from build123d import *

# Parameters (mm, degrees)
F1_DEPTH = 12.7
F3_DEPTH = 12.701
F4_R     = 5.08
F5_DEPTH = 25.4


with BuildPart() as f1:
    # F0 (on Top) → F1 (new body)
    with BuildSketch(Plane.XY):
        Polygon((349.925731, -349.925731), (494.869714, 0), (349.925731, 349.925731), (0, -494.869714), align=None)
    extrude(amount=F1_DEPTH)

    # F2 (on face) → F3 (cut, through all)
    with BuildSketch(Plane.XY.offset(12.7)):
        with BuildLine():
            ThreePointArc((43.288021, -466.629443), (44.712917, -465.460061), (45.248001, -463.696126))
            ThreePointArc((45.248001, -463.696126), (39.433085, -461.93219), (43.288021, -466.629443))
        make_face()
        with BuildLine():
            ThreePointArc((299.347591, -360.566096), (300.772487, -359.396714), (301.307571, -357.632779))
            ThreePointArc((301.307571, -357.632779), (295.492655, -355.868843), (299.347591, -360.566096))
        make_face()
        with BuildLine():
            ThreePointArc((360.566096, -299.347591), (360.746772, -298.751982), (360.807779, -298.132571))
            ThreePointArc((360.807779, -298.132571), (358.252191, -295.018577), (354.699461, -296.917551))
            Line((354.699461, -296.917551), (357.632779, -298.132571))
            Line((357.632779, -298.132571), (360.566096, -299.347591))
        make_face()
        with BuildLine():
            Line((357.632779, -298.132571), (354.699461, -296.917551))
            ThreePointArc((354.699461, -296.917551), (356.417759, -301.065888), (360.566096, -299.347591))
            Line((360.566096, -299.347591), (357.632779, -298.132571))
        make_face()
        with BuildLine():
            ThreePointArc((466.629443, -43.288021), (466.810119, -42.692412), (466.871126, -42.073001))
            ThreePointArc((466.871126, -42.073001), (464.315537, -38.959007), (460.762808, -40.857981))
            Line((460.762808, -40.857981), (463.696126, -42.073001))
            Line((463.696126, -42.073001), (466.629443, -43.288021))
        make_face()
        with BuildLine():
            Line((463.696126, -42.073001), (460.762808, -40.857981))
            ThreePointArc((460.762808, -40.857981), (462.481106, -45.006318), (466.629443, -43.288021))
            Line((466.629443, -43.288021), (463.696126, -42.073001))
        make_face()
        with BuildLine():
            ThreePointArc((466.629443, 43.288021), (460.582132, 41.453589), (466.871126, 42.073001))
            ThreePointArc((466.871126, 42.073001), (466.810119, 42.692412), (466.629443, 43.288021))
        make_face()
        with BuildLine():
            ThreePointArc((360.566096, 299.347591), (354.518786, 297.513159), (360.807779, 298.132571))
            ThreePointArc((360.807779, 298.132571), (360.746772, 298.751982), (360.566096, 299.347591))
        make_face()
    extrude(amount=-F3_DEPTH, mode=Mode.SUBTRACT)

    # F4 (on face) → F5 (cut)
    with BuildSketch(Plane.XY.offset(12.7)):
        with Locations((246.830538, -114.899813)):
            Circle(F4_R)
        with Locations((279.469849, -128.058023)):
            Circle(F4_R)
        with Locations((268.784191, -154.847956)):
            Circle(F4_R)
        with Locations((236.779314, -140.80974)):
            Circle(F4_R)
    extrude(amount=-F5_DEPTH, mode=Mode.SUBTRACT)


solid = f1.part
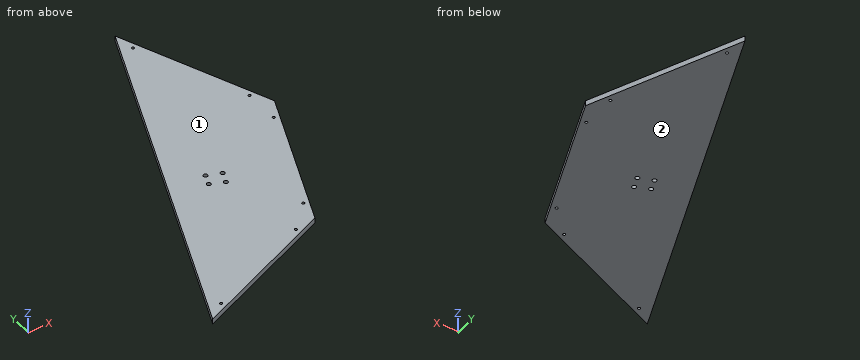
CAD build for the part. Positions are in the model's coordinates, mm. Face numbers are marked on the shaded views. Coordinates: 2 decimals unless noted, no trailing zeros. Order: outer loops, then holes, each group sorted by start corner. A loop starts at its lowest first (then second) coordinate and runs counter-clockwise, first axis right, second up.
Item 1: Band-saw the part on B-B on y = -378. List the corners of the cut face in (x, z), plus the area to 3 significant figures.
Check sheet entries:
outline: (48.41, 0) - (282.15, 0) - (282.15, 12.7) - (48.41, 12.7) - close
area: 2,970 mm2
Item 2: Pin check, flat tips, straight feed: pin 1 Ø6 at (x, y) = (279.47, -128.06) entering from +Z; pin 2 Ø3 at (y, z) = (-385, 5) entering from +X; pin 3 Ø3 at (y, z) = (-52, 10) entering from +X; pin 4 Ø6 at (x, z) = (107, 3) entering from +Y. Stop position of each tip, or through.
Check sheet entries:
pin 1: passes through
pin 2: stops at x = 268.87
pin 3: stops at x = 473.95
pin 4: stops at y = -229.31
Item 3: Drill centre lines: L1, parallel to Y at x = 296, z = 2.75; L2, parallel to Y at x = 29.5, z = 7.75; L3, parallel to Y at x = 178, z = 5.5. Where is each one in solid material? Low to high.
Check sheet entries:
L1: y = -372.26 to -359.98, -355.28 to 219.74
L2: y = -482.65 to -423.65
L3: y = -421.14 to -65.14
Item 4: Band-saw the part on A-A on z = 3. Give the number of separate pieces and of enclosed holes in the cut face, plus the area to 3 significant figures.
Check sheet entries:
separate pieces: 1
enclosed holes: 10
area: 173,000 mm2
Item 5: Two-plate mould, pull along Z, no slides. Class the marked faces 1 and 2: +Z half, -Z half, draft (parallel to the pull), parting line (faces both ways), or undercut.
Check sheet entries:
face 1: +Z half
face 2: -Z half
Item 6: Band-saw the part on C-C on x = 135. List the corners of the cut face in (y, z).
Check sheet entries:
outline: (-438.95, 0) - (-168.95, 0) - (-168.95, 12.7) - (-438.95, 12.7) - close
